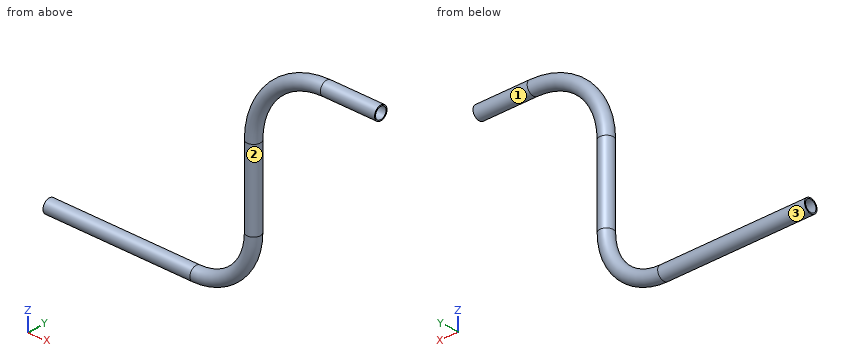
Autodesk Inventor part; units mm, degrees
ref_plane "Work Plane1" through (461.8718, 618.7411, 1.7643) normal (-1, 0, 0) x (0, -1, 0)
ref_plane "YZ Plane" through (0, 0, 0) normal (1, 0, 0) x (0, 1, 0)
ref_plane "XZ Plane" through (0, 0, 0) normal (0, 1, 0) x (-1, 0, 0)
ref_plane "Work Plane1" through (461.8718, 618.7411, 1.7643) normal (-1, 0, 0) x (0, -1, 0)
sketch "Sketch3" plane through (461.8718, 618.7411, 1.7643) normal (-1, 0, 0) x (0, -1, 0)
  circle A0 centre (0, 0) radius 4.7625
  circle A1 centre (0, 0) radius 4.0005
sketch3d "3D Sketch1"
  line L0 (461.8718, 618.7411, 1.7643) -> (424.1819, 618.7411, 1.7643)
  arc A0 (424.1819, 618.7411, 1.7643) -> (373.382, 618.7411, -49.0356) centre (424.1819, 618.7411, -49.0356) ccw
  line L1 (373.382, 618.7411, -49.0356) -> (373.382, 618.7411, -104.3401)
  arc A1 (373.382, 618.7411, -104.3401) -> (333.3821, 618.7411, -144.34) centre (333.3821, 618.7411, -104.3401) ccw
  line L2 (333.3821, 618.7411, -144.34) -> (231.1845, 618.7411, -144.34)
  dimension "d4" = 50.7999
  dimension "d5" = 39.9999
sweep "Sweep1" add profiles "Sketch3" path "3D Sketch1"
equation "\"OD\" = 9.525"
equation "\"t\" = 0.762"
equation "\"L\" = PL"
equation "\"ID\" = 8.001"
equation "\"PL\" = 337.82"
equation "\"Size_Designation\" = 1.2345"
properties material "Copper"
Can you work these out from the model? Positions are in its coordinate system, mm. Face numbers are marked on the shaded views. A direction names the side the tool comes from. Round coordinates to 2 decimals unless told otherwise and drop trailing zeros. Loops run counter-clockwise (first coordinate to the right, second up) from the corner with the lowest first, then second, coordinate; pieces in that order, holes last. Notation, with made-up numbers: (84, 10) - (94, 10) arc R14 cw to (94, 26) - close; hole circle Ø10 at (-27.5, -31.75). An arc over 180 degrees is marked (long way). Use CSV: the item, a comma, the result in double quotes. Start each with the question number.
1) If we section it at B-B on x = 429.5: Write out the boundary of the cut face in (y, z) (1 decimal).
2) For pin 1 Ø5 at (x, z) = (369.5, -107) entering from +Y; pin 2 Ø1.5 at (y, z) = (621, -39.5) entering from +X; pin 3 Ø1 at (x, y) = (341.5, 621.5) entering from +Z, each with a flat end and sliding along its axis, tell me the tip position at first contact or that it passes through.
3) If we section it at C-C on z = -54.5: Write out the boundary of the cut face in (x, y) (1 decimal).
4) If we section it at A-A on y = 619.25: Write out the boundary of the cut face in (x, z), plus the area to 3 significant figures.
5) Please list where these lines run through material, in increasing order: probe 1 along Z at (x, y) = (316, 618.75); probe 2 along X at (y, z) = (618.75, -90.5); probe 3 along X at (y, z) = (622, -59). Write a range as [from, to].
6) For the marked faces 1, 2 and 3, which set-ups out of +Z, -Z, +X, -X, +Y, -Y let a thin tool reach every point of the face, with its end or its side?
Geometry results:
1,outline,"circle Ø9.5 at (618.7, 1.8); hole circle Ø8 at (618.7, 1.8)"
2,pin 1,"stops at y = 623.33"
2,pin 2,"stops at x = 378.94"
2,pin 3,"stops at z = -139.19"
3,outline,"circle Ø9.5 at (373.4, 618.7); hole circle Ø8 at (373.4, 618.7)"
4,outline,"(231.18, -149.08) - (333.38, -149.08) arc R44.74 ccw to (378.12, -104.34) - (378.12, -49.04) arc R46.06 cw to (424.18, -2.97) - (461.87, -2.97) - (461.87, -2.2) - (424.18, -2.2) arc R46.83 ccw to (377.35, -49.04) - (377.35, -104.34) arc R43.97 cw to (333.38, -148.31) - (231.18, -148.31) - close; (231.18, -140.37) - (333.38, -140.37) arc R36.03 ccw to (369.41, -104.34) - (369.41, -49.04) arc R54.77 cw to (424.18, 5.73) - (461.87, 5.73) - (461.87, 6.5) - (424.18, 6.5) arc R55.54 ccw to (368.65, -49.04) - (368.65, -104.34) arc R35.26 cw to (333.38, -139.6) - (231.18, -139.6) - close"
4,area,"518 mm2"
5,probe 1,"z = [-149.1, -148.34], [-140.34, -139.58]"
5,probe 2,"x = [368.62, 369.38], [377.38, 378.14]"
5,probe 3,"x = [369.91, 371.06], [375.7, 376.85]"
6,face 1,"+X"
6,face 2,"none"
6,face 3,"-X"
